Autodesk Inventor part; units mm, degrees
ref_plane "YZ Plane" through (0, 0, 0) normal (1, 0, 0) x (0, 1, 0)
ref_plane "XZ Plane" through (0, 0, 0) normal (0, 1, 0) x (-1, 0, 0)
ref_plane "XY Plane" through (0, 0, 0) normal (0, 0, 1) x (1, 0, 0)
sketch "Sketch1" plane through (0, 0, 0) normal (0, 1, 0) x (-1, 0, 0)
  arc A0 (472.3938, 0) -> (145.9777, 449.2732) centre (0, 0) ccw
  arc A1 (77.994, -240.0408) -> (252.3938, 0) centre (0, 0) ccw
  line L0 (-442.5303, 165.2961) -> (-220.837, 122.2033)
  line L1 (-442.5303, -165.2961) -> (-220.837, -122.2033)
  arc A2 (252.3938, 0) -> (-220.837, 122.2033) centre (0, 0) ccw
  arc A3 (-220.837, -122.2033) -> (77.994, -240.0408) centre (0, 0) ccw
  arc A4 (145.9777, 449.2732) -> (-442.5303, 165.2961) centre (0, 0) ccw
  arc A5 (-442.5303, -165.2961) -> (472.3938, 0) centre (0, 0) ccw
  arc A6 (-218.7278, -117.7184) -> (-218.7278, 117.7184) centre (0, 0) ccw
  arc A7 (-447.907, -162.2663) -> (-447.907, 162.2663) centre (0, 0) ccw
  line L2 (-218.7278, 117.7184) -> (-447.907, 162.2663)
  line L3 (-218.7278, -117.7184) -> (-447.907, -162.2663)
  dimension "d41" = 4
  dimension "d42" = 4
  dimension "d43" = 4
  dimension "d44" = 4
extrude "Extrusion1" add sketch "Sketch1" along normal blind 30
properties part number "Level 1 Edge Banding"
Check sheet for the modelled part. Datum: model origin and axes. Units: mm. A direction names the side the tool comes from. Round coordinates to 2 decimals unless told otherwise and drop trailing zeros. Order: outer loops, then holes, each group sorted by start corner. A loop starts at its lowest first (then second) coordinate and runs counter-clockwise, first axis right, second up. Notation, with made-up numbers: (-32, 36.25) -> (-22, 36.25) arc R26 ccw to (-22, 59.25) -> close; hole circle Ø1 at (-15, -18.5). An arc over 180 degrees is marked (long way). One line per item, written item: value. Start each with the question number.
Q1. Cross-section at A-A (y = 10.5). Record the boundary of the cut face in (x, z).
Q2. Mould release check, pull along Z, two halves, no side actions. Record for faces 1 (the face through (-476.03, 14.79, 18.63)), 2 (the face through (90.32, 14.79, -235.68)), 3 (the face through (-252, 0, 2)): pulls with the +Z half, pulls with the -Z half, needs draft (parallel to the pull), parting line crosses it, or undercut.
Q3. Cross-section at D-D (x = 280). Record the boundary of the cut face in (y, z).
Q4. Set-up check for faces 4 (the face through (-58.59, 14.79, 245.5)), 5 (the face through (-252, 30, 2)), 6 (the face through (331.71, 14.79, -139.68)): record each of +Z, -Z, +X, -X, +Y, -Y from which the full face is reachable in a straight line by a thin tool's end or side.
Q5. Cross-section at C-C (z = -21). Record the boundary of the cut face in (x, y).
Q6. Cross-section at B-B (x = 0). Record the boundary of the cut face in (y, z), and give its area (3 significant figures).
Q7. Thickness scan on line 1 (Z direction, x = 0, y = 10.5); line 2 (X direction, y = 19.5, z = 0); line 3 (Z direction, x = -56.5, y = 19.25). Record the ranges inside material, lowest first.
Q8. Gauge pin test, flat ends, axial feed: pin 1 Ø4 at (x, y) = (-60, 10) entering from -Z; pin 2 Ø1 at (y, z) = (14.5, 213) entering from +X; pin 3 Ø1 at (x, y) = (182.5, 21) entering from +Z. Record the tip position at first contact, or that the pin passes through.
Completed:
1. outline: (218.73, -117.72) arc R248.39 cw (long way) to (218.73, 117.72) -> (447.91, 162.27) arc R476.39 ccw (long way) to (447.91, -162.27) -> close; hole (-472.39, 0) arc R472.39 ccw to (442.53, -165.3) -> (220.84, -122.2) arc R252.39 cw to (-77.99, -240.04) arc R252.39 cw to (-252.39, 0) arc R252.39 cw to (220.84, 122.2) -> (442.53, 165.3) arc R472.39 ccw to (-145.98, 449.27) arc R472.39 ccw to start
2. face 1: parting line crosses it
2. face 2: undercut
2. face 3: needs draft
3. outline: (0, -385.42) -> (30, -385.42) -> (30, -380.47) -> (0, -380.47) -> close; (0, -133.7) -> (30, -133.7) -> (30, -129.63) -> (0, -129.63) -> close; (0, 129.63) -> (30, 129.63) -> (30, 133.7) -> (0, 133.7) -> close; (0, 380.47) -> (30, 380.47) -> (30, 385.42) -> (0, 385.42) -> close
4. face 4: +Y, -Y
4. face 5: +Z, -Z, +X, -X, +Y
4. face 6: +X, +Y, -Y
5. outline: (-475.93, 0) -> (-471.93, 0) -> (-471.93, 30) -> (-475.93, 30) -> close; (-251.52, 0) -> (-247.5, 0) -> (-247.5, 30) -> (-251.52, 30) -> close
6. outline: (0, -476.39) -> (30, -476.39) -> (30, -472.39) -> (0, -472.39) -> close; (0, -252.39) -> (30, -252.39) -> (30, -248.39) -> (0, -248.39) -> close; (0, 248.39) -> (30, 248.39) -> (30, 252.39) -> (0, 252.39) -> close; (0, 472.39) -> (30, 472.39) -> (30, 476.39) -> (0, 476.39) -> close
6. area: 480 mm²
7. line 1: z = -476.39 to -472.39, -252.39 to -248.39, 248.39 to 252.39, 472.39 to 476.39
7. line 2: x = -476.39 to -472.39, -252.39 to -248.39
7. line 3: z = -473.03 to -469, -245.99 to -241.88, 241.88 to 245.99, 469 to 473.03
8. pin 1: stops at z = -472.85
8. pin 2: stops at x = 426.37
8. pin 3: stops at z = 440.26
